The model under review builds one solid part; all positions refer to its coordinate system, in mm. A direction names the side the tool comes from. Give positions to 0.01 mm unless a question says otherwise; leave off trailing zeros. Order: outer loops, then holes, each group sorted by start corner. A loop starts at its lowest first (then second) coordinate and runs counter-clockwise, first axis right, second up. Notation, with made-up numbers: (19, 59) -> (65, 59) arc R35 ccw to (65, 93) -> close; hole circle Ø8 at (52, 12). An arc over 180 degrees is marked (long way). Use one line per item in the form item = value.
```python
from build123d import *

# Parameters (mm, degrees)
SKETCH_1_R      = 2
EXTRUDE_1_DEPTH = 8
SKETCH_2_W      = 4
SKETCH_2_H      = 10
EXTRUDE_2_DEPTH = 8


with BuildPart() as part:
    # 草图1 → 凸台-拉伸1 (new body)
    with BuildSketch(Plane.XY):
        Polygon((-1.831289914, -3), (-1.831289914, 3), (-10.031289914, 3), (-10.031289914, 17), (-14.031289914, 17), (-14.031289914, -3), (-10.031289914, -3), (-10.031289914, -5), (10.031289914, -5), (10.031289914, -3), (14.031289914, -3), (14.031289914, 17), (10.031289914, 17), (10.031289914, 3), (1.831289914, 3), (1.831289914, -3), align=None)
        with Locations((-4.5, 0)):
            Circle(SKETCH_1_R, mode=Mode.SUBTRACT)
        with Locations(Location((4.5, 0, 0), (0, 0, 180))):
            Circle(SKETCH_1_R, mode=Mode.SUBTRACT)
    extrude(amount=EXTRUDE_1_DEPTH)

    # 草图2 → 凸台-拉伸2 (add)
    with BuildSketch(Plane.XY.offset(8)):
        with Locations((-12.031289914, 12)):
            Rectangle(SKETCH_2_W, SKETCH_2_H)
        with Locations((12.031289914, 12)):
            Rectangle(SKETCH_2_W, SKETCH_2_H)
    extrude(amount=EXTRUDE_2_DEPTH)


solid = part.part
```
1. The part is to be moulded in two halves that separate along Y. For faces 1 (the face through (0, -5, 4)), 2 (the face through (-6.4, 1.3, 0)), 3 (the face through (6.1, 1.2, 3.9)), 4 (the face through (-12, 17, 8)), say which applies: +Y half, -Y half, draft (parallel to the pull), parting line (faces both ways), or undercut.
Values:
face_1 = -Y half
face_2 = draft
face_3 = undercut
face_4 = +Y half
2. For pin 1 Ø4.5 at (x, z) = (13, 10) entering from -Y; pin 2 Ø1.1 at (x, z) = (-0.5, 2) entering from +Y; pin 3 Ø0.6 at (y, z) = (-4, 2.5) entering from +X; pin 4 Ø3 at (x, y) = (-4.5, 0) entering from -Z, all flat-tipped, find the tip position at first contact; note any pin that passes through.
Values:
pin_1 = -3
pin_2 = -3
pin_3 = 10.03
pin_4 = through
3. For L1, parallel to X at y = 12, z = 3; L2, parallel to Y at x = -4.5, z = 5.5; L3, parallel to Z at x = -9.25, y = 1, list the stretches that pass through material, from the lowest coordinate up.
Values:
L1 = -14.03 to -10.03, 10.03 to 14.03
L2 = -5 to -2, 2 to 3
L3 = 0 to 8
4. Add section B-B on x = 4.5. Give the boundary of the cut face in (y, z), then the cut area to 3 significant figures.
Values:
outline = (-5, 0) -> (-2, 0) -> (-2, 8) -> (-5, 8) -> close; (2, 0) -> (3, 0) -> (3, 8) -> (2, 8) -> close
area = 32.0 mm^2
5. Add section A-A on y = 4. Give the boundary of the cut face in (x, z), then the cut area to 3 significant figures.
Values:
outline = (-14.03, 0) -> (-10.03, 0) -> (-10.03, 8) -> (-14.03, 8) -> close; (10.03, 0) -> (14.03, 0) -> (14.03, 8) -> (10.03, 8) -> close
area = 64.0 mm^2
6. Tool access review of faces 5 (the face through (-12, 7, 12)), 6 (the face through (-6.1, -1.2, 3.9)), 7 (the face through (10.031, 12, 8)), 8 (the face through (12, -3, 4)), 9 (the face through (-12, -3, 4)): name each direction out of +Z, -Z, +X, -X, +Y, -Y from which nothing blocks a thin tool from reaching the whole face with its end or side.
Values:
face_5 = +Z, +X, -X, -Y
face_6 = +Z, -Z
face_7 = +Z, -Z, +Y
face_8 = +Z, -Z, +X, -Y
face_9 = +Z, -Z, -X, -Y
7. Add section C-C on y = 0. Give the boundary of the cut face in (x, z), then the cut area to 3 significant figures.
Values:
outline = (-14.03, 0) -> (-6.5, 0) -> (-6.5, 8) -> (-14.03, 8) -> close; (-2.5, 0) -> (-1.83, 0) -> (-1.83, 8) -> (-2.5, 8) -> close; (1.83, 0) -> (2.5, 0) -> (2.5, 8) -> (1.83, 8) -> close; (6.5, 0) -> (14.03, 0) -> (14.03, 8) -> (6.5, 8) -> close
area = 131 mm^2
8. Add section D-D on x = 11.25. Give the boundary of the cut face in (y, z).
Values:
outline = (-3, 0) -> (17, 0) -> (17, 16) -> (7, 16) -> (7, 8) -> (-3, 8) -> close
